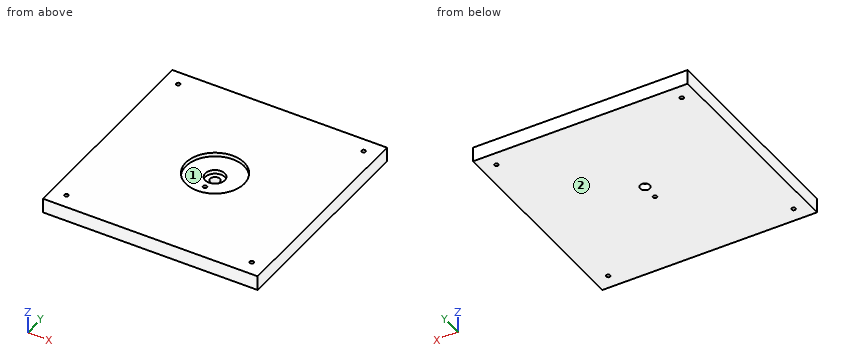
```python
from build123d import *

# Parameters (mm, degrees)
SKETCH2_W           = 279.4
SKETCH2_H           = 279.4
BOSS_EXTRUDE1_DEPTH = 19.05
SKETCH6_R           = 12.7
CUT_EXTRUDE3_DEPTH  = 10.16
SKETCH8_R           = 38.1
CUT_EXTRUDE4_DEPTH  = 5.08
SKETCH9_R           = 6.35
CUT_EXTRUDE5_DEPTH  = 39.37
SKETCH10_R          = 2.54
CUT_EXTRUDE6_DEPTH  = 39.37
SKETCH11_R          = 2.54
CUT_EXTRUDE7_DEPTH  = 36.576


with BuildPart() as part:
    # Sketch2 → Boss-Extrude1 (new body)
    with BuildSketch(Plane.XY):
        Rectangle(SKETCH2_W, SKETCH2_H)
    extrude(amount=BOSS_EXTRUDE1_DEPTH)

    # Sketch6 → Cut-Extrude3 (cut)
    with BuildSketch(Plane.XY.offset(19.05)):
        Circle(SKETCH6_R)
    extrude(amount=-CUT_EXTRUDE3_DEPTH, mode=Mode.SUBTRACT)

    # Sketch8 → Cut-Extrude4 (cut)
    with BuildSketch(Plane.XY.offset(19.05)):
        Circle(SKETCH8_R)
    extrude(amount=-CUT_EXTRUDE4_DEPTH, mode=Mode.SUBTRACT)

    # Sketch9 → Cut-Extrude5 (cut)
    with BuildSketch(Plane.XY.offset(8.89)):
        Circle(SKETCH9_R)
    extrude(amount=-CUT_EXTRUDE5_DEPTH, mode=Mode.SUBTRACT)

    # Sketch10 → Cut-Extrude6 (cut)
    with BuildSketch(Plane.XY.offset(19.05)):
        with Locations((-120.65, -120.65)):
            Circle(SKETCH10_R)
        with Locations((-120.65, 120.65)):
            Circle(SKETCH10_R)
        with Locations((120.65, 120.65)):
            Circle(SKETCH10_R)
        with Locations((120.65, -120.65)):
            Circle(SKETCH10_R)
    extrude(amount=-CUT_EXTRUDE6_DEPTH, mode=Mode.SUBTRACT)

    # Sketch11 → Cut-Extrude7 (cut)
    with BuildSketch(Plane.XY.offset(19.05)):
        with Locations((0, -21.59)):
            Circle(SKETCH11_R)
    extrude(amount=-CUT_EXTRUDE7_DEPTH, mode=Mode.SUBTRACT)


solid = part.part
```
Verification items for the finished model (mm, model axes). Face numbers are marked on the shaded views. Coordinates: 2 decimals unless noted, no trailing zeros. Write each loop counter-clockwise with the first axis right and the second up, starting at its lowest first coordinate (ties: lowest second). Pieces come first, ordered by that corner, then holes. Notation, with made-up numbers: (61, -26.5) - (87, -26.5) arc R10 cw to (87, -17.5) - close; hole circle Ø3 at (-28.75, -25). An arc over 180 degrees is marked (long way). One line per question, with ' | ' between items. Start each with the question number.
1. Draft check along Y on the marked faces 1 and 2. Enter one of: released by +Y, released by -Y, zero draft, split by the parting line, or undercut.
2. Material ranges on line 1 along Y through (x, z) = (-120.65, 10); line 2 along Y through (x, z) = (0, 6); line 3 along Y through (x, z) = (0, 17.2), recorded low to high.
3. Section check A-A (x = -19.5). Enter the section's corners in (y, z).
4. Section check B-B (x = 23.5). Enter the section's corners in (y, z), plus the area to 3 significant figures.
5. Gauge pin test, flat ends, axial feed: P1, Ø10, axis at x = 0, y = 0, coming from the +Z side; P2, Ø12.5, axis at x = -2.5, y = -5.5, coming from the +Z side. Record the tip position at first contact, or that the pin passes through.
Computed values:
1) face 1: undercut | face 2: zero draft
2) line 1: -139.7 to -123.19, -118.11 to 118.11, 123.19 to 139.7 | line 2: -139.7 to -24.13, -19.05 to -6.35, 6.35 to 139.7 | line 3: -139.7 to -38.1, 38.1 to 139.7
3) outline: (-139.7, 0) - (139.7, 0) - (139.7, 19.05) - (32.73, 19.05) - (32.73, 13.97) - (-32.73, 13.97) - (-32.73, 19.05) - (-139.7, 19.05) - close
4) outline: (-139.7, 0) - (139.7, 0) - (139.7, 19.05) - (29.99, 19.05) - (29.99, 13.97) - (-29.99, 13.97) - (-29.99, 19.05) - (-139.7, 19.05) - close | area: 5,020 mm²
5) P1: through | P2: z = 8.89
